CAD build for the part. Positions are in the model's coordinates, mm. A direction names the side the tool comes from. Round coordinates to 2 decimals unless told otherwise and drop trailing zeros. Loops run counter-clockwise (first coordinate to the right, second up) from the corner with the lowest first, then second, coordinate; pieces in that order, holes last.
Autodesk Inventor part; units mm, degrees
ref_plane "YZ Plane" through (0, 0, 0) normal (1, 0, 0) x (0, 1, 0)
ref_plane "XZ Plane" through (0, 0, 0) normal (0, 1, 0) x (-1, 0, 0)
ref_plane "XY Plane" through (0, 0, 0) normal (0, 0, 1) x (1, 0, 0)
sketch "Sketch1" plane through (0, 0, 0) normal (0, 0, 1) x (1, 0, 0)
  line L0 (-12, 22.5) -> (12, 22.5)
  line L1 (12, 22.5) -> (12, -22.5)
  line L2 (12, -22.5) -> (-12, -22.5)
  line L3 (-12, -22.5) -> (-12, 22.5)
  point P0 (0, 0)
  point P1 (12, 0)
  point P2 (0, 22.5)
  dimension "d0" = 24
  dimension "d1" = 45
extrude "Extrusion1" add sketch "Sketch1" along normal blind 31
fillet "Fillet1" radius 3 4 edges at (12, 22.5, 15.5) (-12, 22.5, 15.5) (12, -22.5, 15.5) (-12, -22.5, 15.5)
sketch "Sketch3" plane through (0, 0, 31) normal (0, 0, 1) x (1, 0, 0)
  line L0 (0, -22.5) -> (0, -13.5) construction
  circle A0 centre (0, -13.5) radius 1.5
  point P0 (0, 0)
  dimension "d8" = 9
  dimension "d9" = 3
extrude "Extrusion3" cut sketch "Sketch3" against normal blind 5
sketch "Sketch4" plane through (0, 0, 31) normal (0, 0, 1) x (1, 0, 0)
  circle A0 centre (-9, 19.5) radius 1
  circle A1 centre (9, 19.5) radius 1
  circle A2 centre (-9, -19.5) radius 1
  circle A3 centre (9, -19.5) radius 1
  line L0 (-12, 19.5) -> (-12, -19.5)
  line L1 (9, 22.5) -> (-9, 22.5)
  line L2 (12, -19.5) -> (12, 19.5)
  line L3 (-9, -22.5) -> (9, -22.5)
  point P0 (0, 0)
  dimension "d12" = 2
  dimension "d13" = 3
  dimension "d14" = 3
  dimension "d15" = 3
  dimension "d16" = 3
  dimension "d17" = 3
  dimension "d18" = 3
  dimension "d19" = 3
  dimension "d20" = 3
  dimension "d21" = 2
  dimension "d22" = 2
  dimension "d23" = 2
extrude "Extrusion4" cut sketch "Sketch4" against normal up to surface (31 mm away)
properties part number "herkulex"
Item 1: Mould opens along X. For faces 3 (the cylindrical face through (-9.217, 18.524, 15.717)), 4 (the flat face through (-12, 0, 15)), 5 (the cylindrical face through (11.14, 21.6, 15.72)) say: released by +X, released by -X, zero draft, split by the parting line, or undercut.
Verdict:
face 3: undercut
face 4: released by -X
face 5: released by +X
Item 2: Cut at A-A (z = 15.5). List the corners of the cut face in (x, y).
Verdict:
outline: (-12, -19.5) arc R3 ccw to (-9, -22.5) - (9, -22.5) arc R3 ccw to (12, -19.5) - (12, 19.5) arc R3 ccw to (9, 22.5) - (-9, 22.5) arc R3 ccw to (-12, 19.5) - close; hole circle Ø2 at (-9, -19.5); hole circle Ø2 at (-9, 19.5); hole circle Ø2 at (9, -19.5); hole circle Ø2 at (9, 19.5)
Item 3: Wall check: L1, parallel to Y at x = 9, z = 15; L2, parallel to X at y = 19, z = 20; L3, parallel to Y at x = -9.5, z = 8. Give the ranges that are in metal, low to high.
Verdict:
L1: y = -22.5 to -20.5, -18.5 to 18.5, 20.5 to 22.5
L2: x = -12 to -9.87, -8.13 to 8.13, 9.87 to 12
L3: y = -22.46 to -20.37, -18.63 to 18.63, 20.37 to 22.46
Item 4: Cut at B-B (y = -13.5). List the corners of the cut face in (x, z).
Verdict:
outline: (-12, 0) - (12, 0) - (12, 31) - (1.5, 31) - (1.5, 26) - (-1.5, 26) - (-1.5, 31) - (-12, 31) - close
Item 5: Cut at C-C (z = 27.5). List the corners of the cut face in (x, y).
Verdict:
outline: (-12, -19.5) arc R3 ccw to (-9, -22.5) - (9, -22.5) arc R3 ccw to (12, -19.5) - (12, 19.5) arc R3 ccw to (9, 22.5) - (-9, 22.5) arc R3 ccw to (-12, 19.5) - close; hole circle Ø2 at (-9, -19.5); hole circle Ø2 at (-9, 19.5); hole circle Ø3 at (0, -13.5); hole circle Ø2 at (9, -19.5); hole circle Ø2 at (9, 19.5)
Item 6: 3-axis set-ups, long thin cutter, end or side, ignore diameter. For faces 1 (the flat face through (0, -13, 26)), 2 (the flat face through (0, 0, 0)): which of +Z, -Z, +X, -X, +Y, -Y reach the whole face in a straight line?
Verdict:
face 1: +Z
face 2: -Z, +X, -X, +Y, -Y
Item 7: Flat gauge pins, fed straight in: P1, Ø2.5, axis at x = 0.5, y = -13.5, coming from the +Z side; P2, Ø2.5, axis at x = 0, y = -13.5, coming from the +Z side; P3, Ø1.6, axis at x = -9, y = 19.5, coming from the +Z side. Where does each tip first touch, or does it go through?
Verdict:
P1: stops at z = 31
P2: stops at z = 26
P3: passes through
